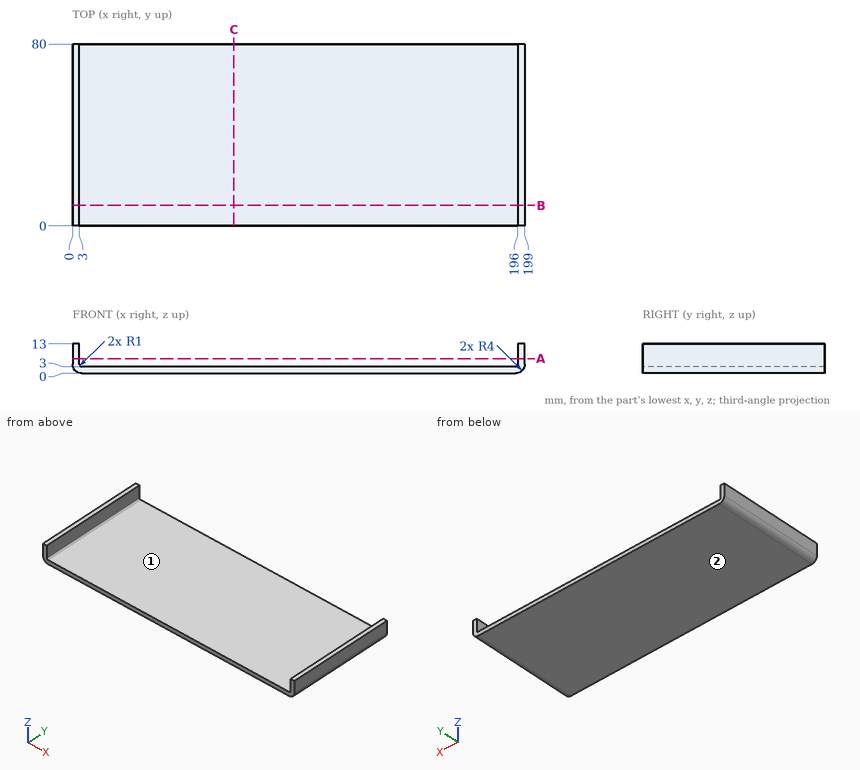
Answer from the drawing. Dimensions are ordinates in mm from the lowest x, y and z of the part. Give positions to 0.01 mm unless a question says otherwise; leave off trailing zeros. Order: outer loops, then holes, each group sorted by start corner. A loop starts at its lowest first (then second) coordinate and runs counter-clockwise, first axis right, second up.
(1) Find section A-A (z = 6.5). Give the vertices of the cut face in (x, y), plus the area to 3 significant figures.
(2) Straight lines are drawn through the part: L1, parallel to X at y = 22, z = 4.75; L2, parallel to Z at x = 98, y = 65; L3, parallel to X at y = 33.5, z = 3.25. For each, find the intervals that lie inside material, in ascending order.
(3) Find section B-B (y = 9). Give the vertices of the cut face in (x, z).
(4) Given pin 1 (8 mm diameter, centred on x = 126.5, y = 50, fed in from -Z); pin 2 (6 mm diameter, centred on x = 86.5, z = 8.5, fed in from -Y); pin 3 (10 mm diameter, centred on x = 64, y = 40, fed in from +Z), each flat-ended and moving along its own axis, determine where each tip first touches the part or whether it passes through.
(5) Find section C-C (x = 71). Give the vertices of the cut face in (y, z), plus the area to 3 significant figures.
(6) For a pull along X with two mould halves and no side action, classify the marked faces 1 and 2 as released by +X, released by -X, zero draft, split by the parting line, or undercut.
Result sheet:
1. outline: (0, 0) - (3, 0) - (3, 80) - (0, 80) - close; (196, 0) - (199, 0) - (199, 80) - (196, 80) - close
1. area: 480 mm2
2. L1: x = 0 to 3, 196 to 199
2. L2: z = 0 to 3
2. L3: x = 0.07 to 3.34, 195.66 to 198.93
3. outline: (0, 4) arc R4 ccw to (4, 0) - (195, 0) arc R4 ccw to (199, 4) - (199, 13) - (196, 13) - (196, 4) arc R1 cw to (195, 3) - (4, 3) arc R1 cw to (3, 4) - (3, 13) - (0, 13) - close
4. pin 1: stops at z = 0
4. pin 2: passes through
4. pin 3: stops at z = 3
5. outline: (0, 0) - (80, 0) - (80, 3) - (0, 3) - close
5. area: 240 mm2
6. face 1: undercut
6. face 2: zero draft
